Verification items for this drawing (mm, ordinates from the low corner). A direction names the side the tool comes from. Round coordinates to 2 decimals unless told otherwise and drop trailing zeros. Order: outer loops, then holes, each group sorted by start corner. A loop starts at its lowest first (then second) coordinate and runs counter-clockwise, first axis right, second up. Notation, with made-up numbers: (77, 44) -> (120, 44) arc R19 ccw to (120, 60) -> close; hole circle Ø6 at (62, -27.5). An arc over 180 degrees is marked (long way). Answer in a Markdown table with one row per item. Add a question column.
1. Access from +Z, -Z, +X, -X, +Y, -Y to the whole of each face (thin tool, end or side, straight path). Record for the marked faces 1 and 2.
2. Sectioned sample at C-C, the plane x = 22.5. Record the boundary of the cut face in (y, z).
3. Sectioned sample at B-B, the plane z = 36.5. Record the boundary of the cut face in (x, y) (1 decimal), then the cut area to 3 significant figures.
4. Depth check by flat-ended pin: P1, Ø5, axis at x = 16.5, z = 27.5, coming from the +Y side; P2, Ø2.5, axis at x = 14, z = 39.5, coming from the +Y side; P3, Ø6, axis at y = 10.5, z = 11, coming from the -X side; P4, Ø3, axis at x = 12.75, z = 38.68, coming from the -Y side. Enter the tip coordinate at first touch or a pass-through.
5. Sectioned sample at D-D, the plane y = 19.25. Record the boundary of the cut face in (x, z), then the cut area to 3 significant figures.
6. Sectioned sample at A-A, the plane x = 12.75. Record the boundary of the cut face in (y, z) (1 decimal), then the cut area to 3 significant figures.
7. Material ranges on L1, parallel to Z at x = 12.75, y = 1.4 (1 decimal); L2, parallel to Z at x = 12.5, y = 4.25 (1 decimal); L3, parallel to Y at x = 10, z = 34.5, recorded low to high. Write a range as from..to.
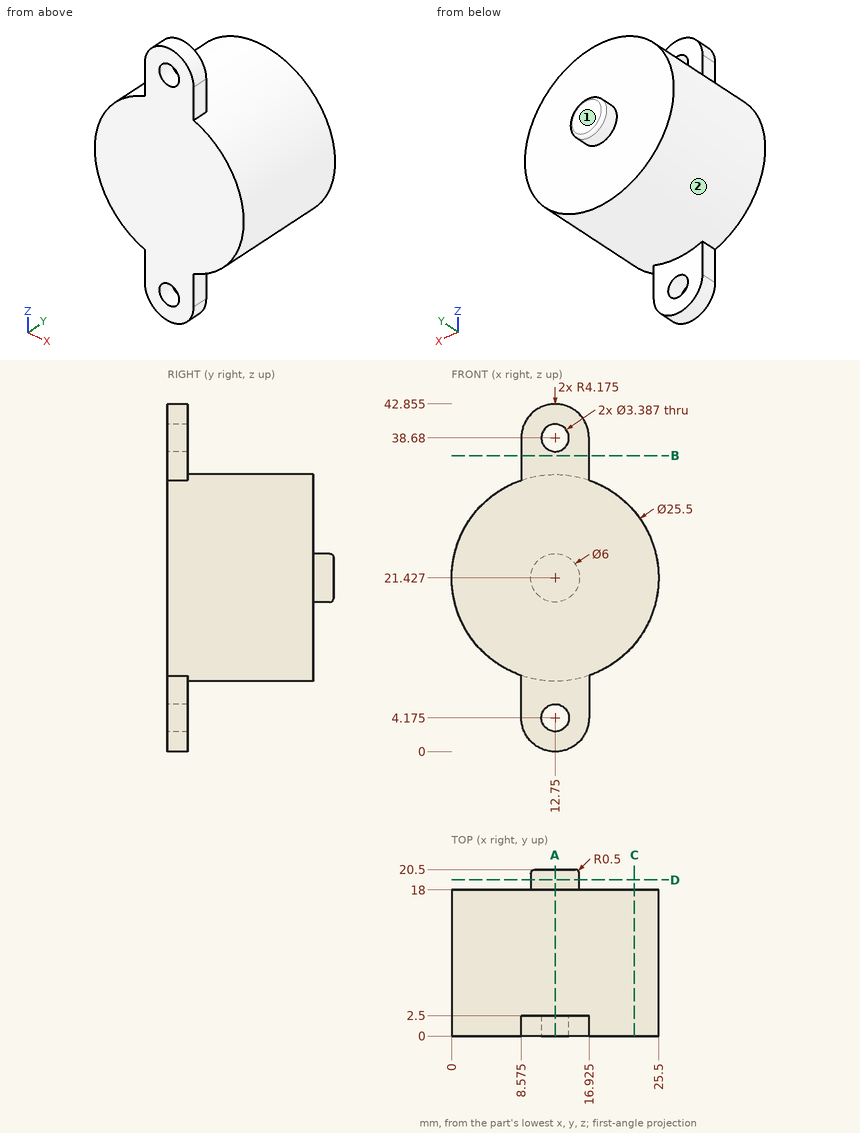
Answer key:
| question | item | result |
|---|---|---|
| 1 | face 1 | +Z, -Z, +X, -X, +Y |
| 1 | face 2 | +Y |
| 2 | outline | (0, 13.21) -> (18, 13.21) -> (18, 29.64) -> (0, 29.64) -> close |
| 3 | outline | (8.6, 0) -> (16.9, 0) -> (16.9, 2.5) -> (8.6, 2.5) -> close |
| 3 | area | 20.9 mm² |
| 4 | P1 | stops at y = 18 |
| 4 | P2 | stops at y = 2.5 |
| 4 | P3 | stops at x = 2.39 |
| 4 | P4 | passes through |
| 5 | outline | circle Ø6 at (12.75, 21.43) |
| 5 | area | 28.3 mm² |
| 6 | outline | (0, 0) -> (2.5, 0) -> (2.5, 2.5) -> (0, 2.5) -> close; (0, 5.9) -> (2.5, 5.9) -> (2.5, 8.7) -> (18, 8.7) -> (18, 18.4) -> (20, 18.4) arc R0.5 ccw to (20.5, 18.9) -> (20.5, 23.9) arc R0.5 ccw to (20, 24.4) -> (18, 24.4) -> (18, 34.2) -> (2.5, 34.2) -> (2.5, 37) -> (0, 37) -> close; (0, 40.4) -> (2.5, 40.4) -> (2.5, 42.9) -> (0, 42.9) -> close |
| 6 | area | 500 mm² |
| 7 | L1 | z = 0..2.5, 5.9..37, 40.4..42.9 |
| 7 | L2 | z = 8.7..34.2 |
| 7 | L3 | y = 0..2.5 |
